Here's the drawing with two shaded views (mm, measured from the low corner). I have some questions. A direction names the side the tool comes from. Round coordinates to 2 decimals unless told otherwise and drop trailing zeros. Order: outer loops, then holes, each group sorted by start corner. A loop starts at its lowest first (then second) coordinate and runs counter-clockwise, first axis right, second up.
Q1. Will these pins go through, and if not, where does the flat tip stop? P1, Ø11, axis at x = 71, y = 14.5, coming from the -Z side; P2, Ø8, axis at x = 135, z = 15, coming from the +Y side; P3, Ø5, axis at x = 130, z = 15, coming from the +Y side; P4, Ø2, axis at x = 91.5, z = 7.5, coming from the -Y side.
Q2. If we section it at A-A (z = 15): Please give me the cut outline in (x, y), plus the area to 3 significant figures.
Q3. If we section it at C-C (x = 70): Please give me the cut outline in (y, z).
Q4. If we section it at B-B (x = 135): Please give me the cut outline in (y, z), plus the area to 3 significant figures.
Q5. For the marked faces 1 and 2, which set-ups out of +Z, -Z, +X, -X, +Y, -Y let a thin tool reach every point of the face, with its end or its side?
Q6. If I drill on line 1 (X direction, y = 27.75, z = 13); line 2 (Y direction, x = 79, z = 10); line 3 (Z direction, x = 28.5, y = 12.5), over which ranges is the centre line in solid material (lowest first)?
Q7. If we section it at D-D (y = 17.5): Please give me the cut outline in (x, z).
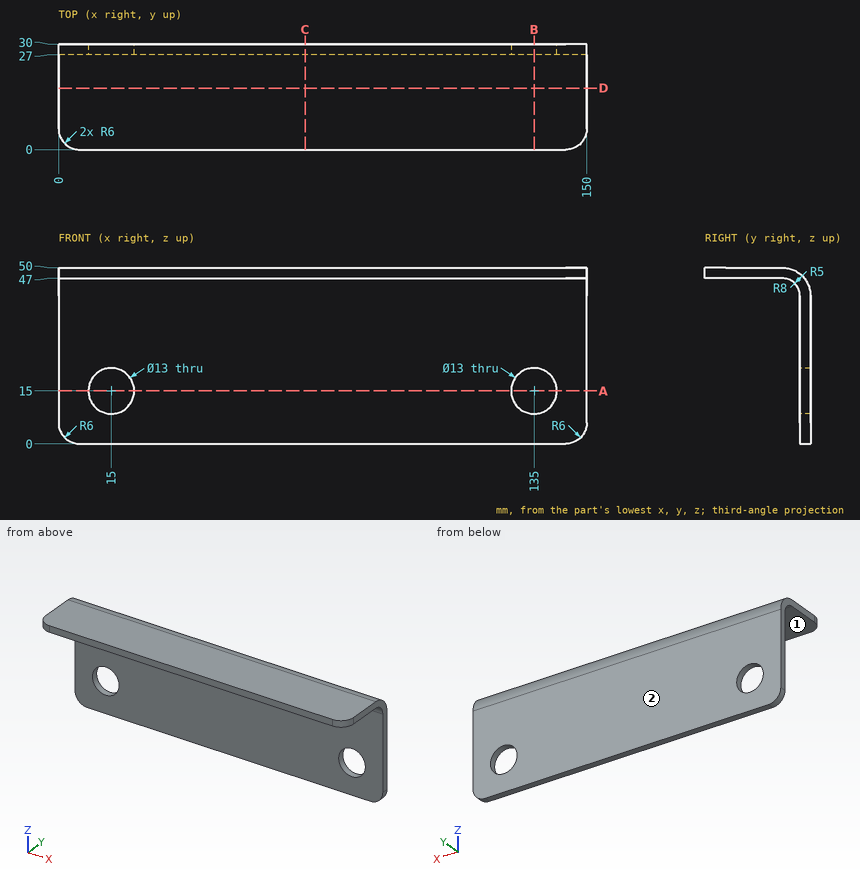
Solution:
1. P1: stops at z = 47
1. P2: passes through
1. P3: stops at y = 30
1. P4: stops at y = 27
2. outline: (0, 27) - (8.5, 27) - (8.5, 30) - (0, 30) - close; (21.5, 27) - (128.5, 27) - (128.5, 30) - (21.5, 30) - close; (141.5, 27) - (150, 27) - (150, 30) - (141.5, 30) - close
2. area: 372 mm2
3. outline: (0, 47) - (22, 47) arc R5 cw to (27, 42) - (27, 0) - (30, 0) - (30, 42) arc R8 ccw to (22, 50) - (0, 50) - close
4. outline: (0, 47) - (22, 47) arc R5 cw to (27, 42) - (27, 21.5) - (30, 21.5) - (30, 42) arc R8 ccw to (22, 50) - (0, 50) - close; (27, 0) - (30, 0) - (30, 8.5) - (27, 8.5) - close
4. area: 184 mm2
5. face 1: -Z, +X, -X, -Y
5. face 2: +Z, -Z, +X, -X, +Y
6. line 1: x = 0 to 8.82, 21.18 to 128.82, 141.18 to 150
6. line 2: y = 27 to 30
6. line 3: z = 47 to 50
7. outline: (0, 47) - (150, 47) - (150, 50) - (0, 50) - close
